```python
from build123d import *

# Parameters (mm, degrees)
SKETCH2_R           = 145
SKETCH2_R_2         = 105
BOSS_EXTRUDE1_START = -50
SKETCH4_W           = 360
SKETCH4_H           = 360
SKETCH4_R           = 145
BOSS_EXTRUDE1_DEPTH = 50
CUT_EXTRUDE1_DEPTH  = 10
CUT_EXTRUDE2_REACH  = 707.355
SKETCH6_R           = 15
CIRPATTERN1_COUNT   = 4
FILLET1_R           = 20
FILLET2_R           = 10
CHAMFER1_SIZE       = 10
SKETCH7_W           = 360
SKETCH7_H           = 360
SKETCH7_R           = 145
BOSS_EXTRUDE2_DEPTH = 50
CUT_EXTRUDE3_DEPTH  = 10
CUT_EXTRUDE4_REACH  = 848.699
SKETCH9_R           = 15
CIRPATTERN3_COUNT   = 4
CHAMFER2_SIZE       = 10
FILLET4_R           = 10


with BuildPart() as part:
    # Sweep-Thin1: sweep along a path in Sketch1
    with BuildLine(Plane.XY) as sweep_thin1_path:
        Line((0, 0), (-150, 0))
        ThreePointArc((-150, 0), (-333.847763109, 76.152236891), (-410, 260))
        Line((-410, 260), (-410, 410))
    # Sketch2 → Sweep-Thin1 (sweep)
    with BuildSketch(Plane(origin=(0, 0, 0), x_dir=(0, 0, -1), z_dir=(1, 0, 0))):
        Circle(SKETCH2_R)
        Circle(SKETCH2_R_2, mode=Mode.SUBTRACT)
    sweep(path=sweep_thin1_path.line)

    # Sketch4 → Boss-Extrude1 (add)
    with BuildSketch(Plane(origin=(0, 0, 0), x_dir=(0, 0, -1), z_dir=(1, 0, 0)).offset(BOSS_EXTRUDE1_START)):
        Rectangle(SKETCH4_W, SKETCH4_H)
        with Locations(Location((0, 0, 0), (0, 0, 270))):
            Circle(SKETCH4_R, mode=Mode.SUBTRACT)
    extrude(amount=BOSS_EXTRUDE1_DEPTH)

    # Sketch5 → Cut-Extrude1 (cut)
    with BuildSketch(Plane(origin=(0, 0, 0), x_dir=(0, 0, -1), z_dir=(1, 0, 0))):
        with BuildLine():
            Line((-130, 100), (-130, 130))
            Line((-130, 130), (-100, 130))
            ThreePointArc((-100, 130), (-151.213203436, 151.213203436), (-130, 100))
        make_face()
        with BuildLine():
            Line((-100, 130), (-130, 130))
            Line((-130, 130), (-130, 100))
            ThreePointArc((-130, 100), (-108.786796564, 108.786796564), (-100, 130))
        make_face()
    cut_extrude1 = extrude(amount=-CUT_EXTRUDE1_DEPTH, mode=Mode.SUBTRACT)

    # Sketch6 → Cut-Extrude2 (cut, up to next)
    with BuildSketch(Plane(origin=(-10, 0, 0), x_dir=(0, 0, -1), z_dir=(1, 0, 0)), mode=Mode.PRIVATE) as cut_extrude2_sk1:
        with Locations((-130, 130)):
            Circle(SKETCH6_R)
    cut_extrude2_tool1 = extrude(cut_extrude2_sk1.sketch, amount=-CUT_EXTRUDE2_REACH, mode=Mode.PRIVATE) & part.part
    cut_extrude2 = cut_extrude2_tool1.solids().sort_by_distance((-10, 130, 130))[0]
    add(cut_extrude2, mode=Mode.SUBTRACT)

    # CirPattern1: Cut-Extrude1, Cut-Extrude2 ×4 about axis
    cirpattern1_axis = Axis((0, 0, 0), (1, 0, 0))
    add([cut_extrude1.rotate(cirpattern1_axis, i * 360 / CIRPATTERN1_COUNT) for i in range(1, CIRPATTERN1_COUNT)], mode=Mode.SUBTRACT)
    add([cut_extrude2.rotate(cirpattern1_axis, i * 360 / CIRPATTERN1_COUNT) for i in range(1, CIRPATTERN1_COUNT)], mode=Mode.SUBTRACT)

    # Fillet1
    fillet1_edges = [part.edges().sort_by_distance(p)[0] for p in [
        (-25, 180, -180),
        (-25, -180, -180),
        (-25, -180, 180),
        (-25, 180, 180),
    ]]
    fillet(fillet1_edges, radius=FILLET1_R)

    # Fillet2
    fillet2_edges = [part.edges().sort_by_distance(p)[0] for p in [
        (-50, 0, 145),
    ]]
    fillet(fillet2_edges, radius=FILLET2_R)

    # Chamfer1
    chamfer1_edges = [part.edges().sort_by_distance(p)[0] for p in [
        (0, 0, 105),
    ]]
    chamfer(chamfer1_edges, length=CHAMFER1_SIZE)

    # Sketch7 → Boss-Extrude2 (add)
    with BuildSketch(Plane(origin=(0, 410, 0), x_dir=(1, 0, 0), z_dir=(0, 1, 0))):
        with Locations((-410, 0)):
            Rectangle(SKETCH7_W, SKETCH7_H)
        with Locations(Location((-410, 0, 0), (0, 0, 270))):
            Circle(SKETCH7_R, mode=Mode.SUBTRACT)
    extrude(amount=-BOSS_EXTRUDE2_DEPTH)

    # Sketch8 → Cut-Extrude3 (cut)
    with BuildSketch(Plane(origin=(0, 410, 0), x_dir=(1, 0, 0), z_dir=(0, 1, 0))):
        with BuildLine():
            Line((-540, 100), (-540, 130))
            Line((-540, 130), (-510, 130))
            ThreePointArc((-510, 130), (-561.213203436, 151.213203436), (-540, 100))
        make_face()
        with BuildLine():
            Line((-510, 130), (-540, 130))
            Line((-540, 130), (-540, 100))
            ThreePointArc((-540, 100), (-518.786796564, 108.786796564), (-510, 130))
        make_face()
    cut_extrude3 = extrude(amount=-CUT_EXTRUDE3_DEPTH, mode=Mode.SUBTRACT)

    # Sketch9 → Cut-Extrude4 (cut, up to next)
    with BuildSketch(Plane(origin=(0, 400, 0), x_dir=(1, 0, 0), z_dir=(0, 1, 0)), mode=Mode.PRIVATE) as cut_extrude4_sk1:
        with Locations(Location((-540, 130, 0), (0, 0, 270))):
            Circle(SKETCH9_R)
    cut_extrude4_tool1 = extrude(cut_extrude4_sk1.sketch, amount=-CUT_EXTRUDE4_REACH, mode=Mode.PRIVATE) & part.part
    cut_extrude4 = cut_extrude4_tool1.solids().sort_by_distance((-540, 400, -130))[0]
    add(cut_extrude4, mode=Mode.SUBTRACT)

    # CirPattern3: Cut-Extrude3, Cut-Extrude4 ×4 about axis
    cirpattern3_axis = Axis((-410, 0, 0), (0, 1, 0))
    add([cut_extrude3.rotate(cirpattern3_axis, i * 360 / CIRPATTERN3_COUNT) for i in range(1, CIRPATTERN3_COUNT)], mode=Mode.SUBTRACT)
    add([cut_extrude4.rotate(cirpattern3_axis, i * 360 / CIRPATTERN3_COUNT) for i in range(1, CIRPATTERN3_COUNT)], mode=Mode.SUBTRACT)

    # Chamfer2
    chamfer2_edges = [part.edges().sort_by_distance(p)[0] for p in [
        (-410, 410, 105),
    ]]
    chamfer(chamfer2_edges, length=CHAMFER2_SIZE)

    # Fillet4
    fillet4_edges = [part.edges().sort_by_distance(p)[0] for p in [
        (-410, 360, 145),
    ]]
    fillet(fillet4_edges, radius=FILLET4_R)


solid = part.part
```
The listing builds one solid part. Answer for the finished solid, in the listing's coordinates (mm). A direction names the side the tool comes from. Give positions to 0.01 mm unless a question says otherwise; leave off trailing zeros. Write each loop counter-clockwise with the first axis right and the second up, starting at its lowest first coordinate (ties: lowest second). Pieces come first, ordered by that corner, then holes. Notation, with made-up numbers: M 16.5,14 L 32.5,14 A4 cw 32.5,20 Z; hole C -4,-5 d9. An arc over 180 degrees is marked long. Write each question's results on one line, items separated by ' | '.
Q1. Section B-B, the plane y = 309.5 is taken. Write down the section's boundary in (x, z).
Output values:
outline: C -410,0 d290; hole C -410,0 d210
Q2. Consider L1, parallel to Y at x = -7, z = -130; L2, parallel to Z at x = -280, y = 378.5. Determine where each line is inside the solid, lowest interval first. Write a range as from..to.
Output values:
L1: -180..-160, -100..100, 160..180 | L2: -180..-145, -115..115, 145..180
Q3. Flat-ended cylindrical pins translate along their axes: P1, Ø6, axis at x = -404, z = 1, coming from the -Y side; P2, Ø3, axis at y = 268.5, z = 57, coming from the -X side; P3, Ø4, axis at y = 36.5, z = 74, coming from the -X side; P4, Ø2, axis at y = 174.5, z = 24.5, coming from the +X side. Find the tip coordinate at first contact, or state that the pin passes through.
Output values:
P1: y = -57.84 | P2: x = -543.96 | P3: x = -465.13 | P4: x = 0
Q4. A tool of negligible diameter and unlimited length cuts with its end or side. For faces 4 (the flat face through (-50, 3, -157)), 5 (the cylindrical face through (-292.65, 380.28, 121.94)), 6 (the cylindrical face through (-24.65, 173.986, 174.297)), 7 (the flat face through (-10, -144, 124)), from which of +Z, -Z, +X, -X, +Y, -Y can it reach the whole face along a straight path? Write none if from no direction.
Output values:
face 4: none | face 5: +Y | face 6: +Z, +X, -X, +Y | face 7: +X
Q5. For a pull along X with two mould halves and no side action, classify faces 1 (the flat face through (-286, 400, -144)), 2 (the cylindrical face through (-532.265, 305.63, -77.951)), 3 (the flat face through (-230, 385, 3)) as released by +X, released by -X, zero draft, split by the parting line, or undercut.
Output values:
face 1: undercut | face 2: split by the parting line | face 3: released by +X
